Design review of the part built by this model. Coordinates are the model's own, in mm. A direction names the side the tool comes from. Give positions to 0.01 mm unless a question says otherwise; leave off trailing zeros. Order: outer loops, then holes, each group sorted by start corner. A loop starts at its lowest first (then second) coordinate and runs counter-clockwise, first axis right, second up.
```python
from build123d import *

# Parameters (mm, degrees)
F1_DEPTH = 254
F2_W     = 85.141710937
F2_H     = 17.5291653723
F3_DEPTH = 292.8777724


# Not quite as in the source:
# - an extrude ends at something that could not be found from the text; its depth is read off the source's solid


with BuildPart() as f1:
    # F0 (on Front) → F1 (new body)
    with BuildSketch(Plane.XZ):
        with BuildLine():
            Line((52.2444248199, 18.3139387518), (-52.2444248199, 18.3139387518))
            ThreePointArc((-52.2444248199, 18.3139387518), (-70.5583635718, 0), (-52.2444248199, -18.3139387518))
            Line((-52.2444248199, -18.3139387518), (52.2444248199, -18.3139387518))
            ThreePointArc((52.2444248199, -18.3139387518), (70.5583635718, 0), (52.2444248199, 18.3139387518))
        make_face()
    extrude(amount=F1_DEPTH)

    # F2 (on Front) → F3 (join, through all)
    with BuildSketch(Plane.XZ):
        Rectangle(F2_W, F2_H)
    extrude(amount=-F3_DEPTH)


solid = f1.part
```
1. For line 1 along Y through (x, z) = (-22.5, 16); line 2 along X through (y, z) = (225, 3); line 3 along Z through (x, y) = (29, 153), list the stretches that pass through material, from the lowest coordinate up.
Recorded:
line 1: y = -254 to 0
line 2: x = -42.57 to 42.57
line 3: z = -8.76 to 8.76
2. Take a section at B-B (x = -25). State the section outline as (y, z) points.
Recorded:
outline: (-254, -18.31) - (0, -18.31) - (0, -8.76) - (292.88, -8.76) - (292.88, 8.76) - (0, 8.76) - (0, 18.31) - (-254, 18.31) - close
3. Take a section at A-A (z = 0). State the section outline as (x, y) points.
Recorded:
outline: (-70.56, -254) - (70.56, -254) - (70.56, 0) - (42.57, 0) - (42.57, 292.88) - (-42.57, 292.88) - (-42.57, 0) - (-70.56, 0) - close
4. Take a section at C-C (y = -87.5). State the section outline as (x, z) points.
Recorded:
outline: (-52.24, -18.31) - (52.24, -18.31) arc R18.31 ccw to (52.24, 18.31) - (-52.24, 18.31) arc R18.31 ccw to start
5. Take a section at D-D (y = 37.5). State the section outline as (x, z) points, then the cut area to 3 significant figures.
Recorded:
outline: (-42.57, -8.76) - (42.57, -8.76) - (42.57, 8.76) - (-42.57, 8.76) - close
area: 1,490 mm2
6. Machinability: for faces 1 (the face through (-1, 144, 8.765)), 2 (the face through (42.571, 144, 0)), 3 (the face through (-42.571, 144, 0)), which of the approach directions +Z, -Z, +X, -X, +Y, -Y give a long, thin tool a straight path to every point of the face, cutting with its end or side? Answer none if there is none.
Recorded:
face 1: +Z, +X, -X, +Y
face 2: +Z, -Z, +X, +Y
face 3: +Z, -Z, -X, +Y
7. For pin 1 (4 mm diameter, centred on x = 51.5, z = -2.5, fed in from +Y); pin 2 (14 mm diameter, centred on y = 79, z = -3.5, fed in from -X); pin 3 (19.5 mm diameter, centred on y = 79.5, z = 0.5, fed in from +X), all flat-tipped, find the tip position at first contact; note any pin that passes through.
Recorded:
pin 1: stops at y = 0
pin 2: stops at x = -42.57
pin 3: stops at x = 42.57
